The listing builds one solid part. Answer for the finished solid, in the listing's coordinates (mm). Face numbers are marked on the shaded views. A direction names the side the tool comes from. Coordinates: 2 decimals unless noted, no trailing zeros. Loops run counter-clockwise (first coordinate to the right, second up) from the corner with the lowest first, then second, coordinate; pieces in that order, holes last. Notation, with made-up numbers: (76, -0.75) - (101, -0.75) arc R10 ccw to (101, 11.25) - close; hole circle Ø6 at (-8, 30). An arc over 180 degrees is marked (long way). Write each question's results on one line, items separated by ' | '. Start each with the question number.
(1) Find section B-B on x = 11. Determine the outline of the cut face in (y, z).
(2) For the marked faces 1, 2, 3 and 4, determine the directions among +Z, -Z, +X, -X, +Y, -Y from which every point of the face is accessible in a straight line to the end or side of a thin tool.
(3) Consider line 1 (X direction, y = 5.75, z = -30); line 2 (Z direction, x = 4, y = 2.5); line 3 (X direction, y = -51, z = -11.5). Determine where each line is inside the solid, lowest interval first. Write a range as from..to.
(4) Find section C-C on y = -13.5. Determine the outline of the cut face in (x, z).
(5) Find section A-A on x = 65. Determine the outline of the cut face in (y, z).
(6) Given pin 1 Ø11.5 at (x, y) = (56, -73) entering from -Z; pin 2 Ø4.5 at (x, y) = (50, -78) entering from +Z; pin 3 Ø12 at (y, z) = (-16, -18) entering from +X, each flat-ended and moving along its own axis, determine where each tip first touches the part or whether it passes through.
from build123d import *

# Parameters (mm, degrees)
SKETCH_1_W                   = 33
SKETCH_1_H                   = 40
EXTRUDE_1_DEPTH              = 10
EXTRUDE_2_DEPTH              = 10
SKETCH_3_W                   = 27
SKETCH_3_H                   = 14.5
EXTRUDE_3_DEPTH              = 28.5
CUT_EXTRUDE_1_DEPTH          = 15
CUT_EXTRUDE_2_REACH          = 116.016
EXTRUDE_4_REACH              = 116.016
EXTRUDE_5_REACH              = 116.016
HOLE_WIZARD_M3_1_D           = 3.4
HOLE_WIZARD_M3_1_CSINK_D     = 6.3
HOLE_WIZARD_M3_1_CSINK_ANGLE = 90
OTHER_START                  = 35
OTHER_1_OUTLINE_R            = 4.05
OTHER_1_DEPTH                = 8


# Read off the part's stored shape, not the designer's step: 高级异型孔1
with BuildPart() as part:
    # 草图1 → 凸台-拉伸1 (new body)
    with BuildSketch(Plane(origin=(0, 0, 0), x_dir=(1, 0, 0), z_dir=(0, 1, 0))):
        with Locations((16.5, 20)):
            Rectangle(SKETCH_1_W, SKETCH_1_H)
    extrude(amount=EXTRUDE_1_DEPTH)

    # 草图2 → 凸台-拉伸2 (add)
    with BuildSketch(Plane(origin=(33, 0, 0), x_dir=(0, 0, -1), z_dir=(1, 0, 0))):
        Polygon((0, 0), (6.5, -67.75), (6.5, -82.25), (33.5, -82.25), (33.5, -67.75), (40, 0), (40, 10), (0, 10), align=None)
    extrude(amount=EXTRUDE_2_DEPTH)

    # 草图3 → 凸台-拉伸3 (add)
    with BuildSketch(Plane(origin=(43, 0, 0), x_dir=(0, 0, -1), z_dir=(1, 0, 0))):
        with Locations((20, -75)):
            Rectangle(SKETCH_3_W, SKETCH_3_H)
    extrude(amount=EXTRUDE_3_DEPTH)

    # 草图4 → 切除-拉伸1 (cut)
    with BuildSketch(Plane.ZY.offset(-71.5)):
        with BuildLine():
            Line((-6.5, -75.5), (-6.5, -73.75))
            Line((-6.5, -73.75), (-33.5, -73.75))
            Line((-33.5, -73.75), (-33.5, -75.5))
            ThreePointArc((-33.5, -75.5), (-32.75, -74.75), (-32, -75.5))
            ThreePointArc((-32, -75.5), (-31.25, -76.25), (-30.5, -75.5))
            ThreePointArc((-30.5, -75.5), (-29.75, -74.75), (-29, -75.5))
            ThreePointArc((-29, -75.5), (-28.25, -76.25), (-27.5, -75.5))
            ThreePointArc((-27.5, -75.5), (-26.75, -74.75), (-26, -75.5))
            ThreePointArc((-26, -75.5), (-25.25, -76.25), (-24.5, -75.5))
            ThreePointArc((-24.5, -75.5), (-23.75, -74.75), (-23, -75.5))
            ThreePointArc((-23, -75.5), (-22.25, -76.25), (-21.5, -75.5))
            ThreePointArc((-21.5, -75.5), (-21.280330086, -74.969669914), (-20.75, -74.75))
            Line((-20.75, -74.75), (-19.25, -74.75))
            ThreePointArc((-19.25, -74.75), (-18.719669914, -74.969669914), (-18.5, -75.5))
            ThreePointArc((-18.5, -75.5), (-17.75, -76.25), (-17, -75.5))
            ThreePointArc((-17, -75.5), (-16.25, -74.75), (-15.5, -75.5))
            ThreePointArc((-15.5, -75.5), (-14.75, -76.25), (-14, -75.5))
            ThreePointArc((-14, -75.5), (-13.25, -74.75), (-12.5, -75.5))
            ThreePointArc((-12.5, -75.5), (-11.75, -76.25), (-11, -75.5))
            ThreePointArc((-11, -75.5), (-10.25, -74.75), (-9.5, -75.5))
            ThreePointArc((-9.5, -75.5), (-8.75, -76.25), (-8, -75.5))
            ThreePointArc((-8, -75.5), (-7.25, -74.75), (-6.5, -75.5))
        make_face()
    extrude(amount=CUT_EXTRUDE_1_DEPTH, mode=Mode.SUBTRACT)

    # 草图5 → 切除-拉伸2 (cut, up to next)
    with BuildSketch(Plane.XY.offset(-6.5), mode=Mode.PRIVATE) as cut_extrude_2_sk1:
        Polygon((33, -82.25), (49.121822718, -82.25), (33, -67.75), align=None)
    cut_extrude_2_tool1 = extrude(cut_extrude_2_sk1.sketch, amount=-CUT_EXTRUDE_2_REACH, mode=Mode.PRIVATE) & part.part
    add(cut_extrude_2_tool1.solids().sort_by_distance((38.373941, -77.416667, -6.5))[0], mode=Mode.SUBTRACT)

    # 凸台-拉伸4: up to this plane
    extrude_4_end = Plane(origin=(43, -67.75, -33.5), z_dir=(0, 0.09550243214662471, 0.9954291966052028))
    # 草图6 → 凸台-拉伸4 (add, up to the surface)
    with BuildSketch(Plane.XY.offset(-6.5), mode=Mode.PRIVATE) as extrude_4_sk1:
        Polygon((43, -57.242064668), (43, -67.75), (54.683246246, -67.75), align=None)
    extrude_4_tool1 = split(extrude(extrude_4_sk1.sketch, amount=-EXTRUDE_4_REACH, mode=Mode.PRIVATE), bisect_by=extrude_4_end, keep=Keep.BOTH, mode=Mode.PRIVATE)
    add(extrude_4_tool1.solids().sort_by_distance((46.894415, -64.247355, -6.5))[0])

    # 凸台-拉伸5: up to this face of the body (flat: up to its plane)
    extrude_5_end = Plane(part.part.faces().sort_by_distance((38, -33.875, -3.25))[0])
    # 草图6<2> → 凸台-拉伸5 (add, up to the picked face)
    with BuildSketch(Plane.XY.offset(-6.5), mode=Mode.PRIVATE) as extrude_5_sk1:
        Polygon((43, -57.242064668), (43, -67.75), (54.683246246, -67.75), align=None)
    extrude_5_tool1 = split(extrude(extrude_5_sk1.sketch, amount=EXTRUDE_5_REACH, mode=Mode.PRIVATE), bisect_by=extrude_5_end, keep=Keep.BOTH, mode=Mode.PRIVATE)
    add(extrude_5_tool1.solids().sort_by(Axis((46.894415, -64.247355, -6.5), (0, 0, 1)))[0])

    # M3 平头机械螺钉的锥形沉头孔1 (through all)
    with Locations(Plane(origin=(0, 10, 0), x_dir=(1, 0, 0), z_dir=(0, 1, 0))):
        with Locations((29, 30), (4, 30), (4, 10), (29, 10)):
            CounterSinkHole(HOLE_WIZARD_M3_1_D / 2, HOLE_WIZARD_M3_1_CSINK_D / 2, counter_sink_angle=HOLE_WIZARD_M3_1_CSINK_ANGLE)

    # 高级异型孔1 outline → 高级异型孔1 (cut)
    with BuildSketch(Plane.YZ.offset(OTHER_START)):
        with Locations((-20, -20)):
            Circle(OTHER_1_OUTLINE_R)
    extrude(amount=OTHER_1_DEPTH, mode=Mode.SUBTRACT)


solid = part.part
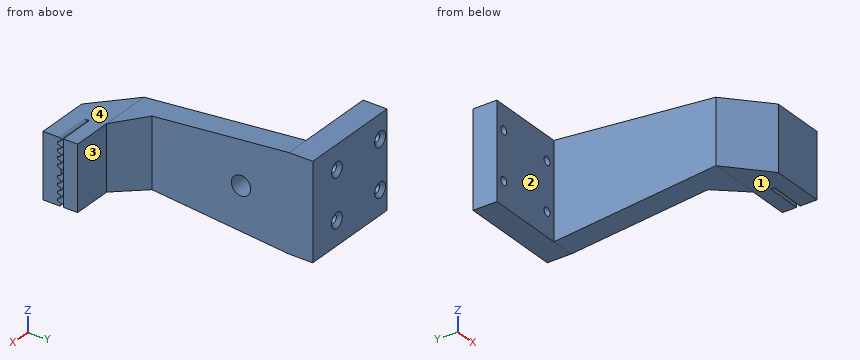
Values:
1) outline: (0, -40) - (10, -40) - (10, 0) - (0, 0) - close
2) face 1: -Z, +X, -X, -Y | face 2: +Z, -Z, -X, -Y | face 3: +Z, -Z, +X, +Y | face 4: +Z, +X, -X, -Y
3) line 1: x = 0..2.3, 5.7..27.3, 30.7..43 | line 2: z = -40..-31.7, -28.3..-11.7, -8.3..0 | line 3: x = 33..43
4) outline: (33, -38.7) - (43, -38.7) - (43, -1.3) - (33, -1.3) - close
5) outline: (-82.25, -33.5) - (-75.5, -33.5) arc R0.75 ccw to (-75.5, -32) arc R0.75 cw to (-75.5, -30.5) arc R0.75 ccw to (-75.5, -29) arc R0.75 cw to (-75.5, -27.5) arc R0.75 ccw to (-75.5, -26) arc R0.75 cw to (-75.5, -24.5) arc R0.75 ccw to (-75.5, -23) arc R0.75 cw to (-75.5, -21.5) arc R0.75 ccw to (-74.75, -20.75) - (-74.75, -19.25) arc R0.75 ccw to (-75.5, -18.5) arc R0.75 cw to (-75.5, -17) arc R0.75 ccw to (-75.5, -15.5) arc R0.75 cw to (-75.5, -14) arc R0.75 ccw to (-75.5, -12.5) arc R0.75 cw to (-75.5, -11) arc R0.75 ccw to (-75.5, -9.5) arc R0.75 cw to (-75.5, -8) arc R0.75 ccw to (-75.5, -6.5) - (-82.25, -6.5) - close; (-73.75, -33.5) - (-67.75, -33.5) - (-67.75, -6.5) - (-73.75, -6.5) - close
6) pin 1: stops at z = -33.53 | pin 2: stops at z = -6.5 | pin 3: stops at x = 43
